```python
from build123d import *

# Parameters (mm, degrees)
SKETCH1_W                     = 42
SKETCH1_H                     = 20
BOSS_EXTRUDE1_DEPTH           = 5
SKETCH2_W                     = 21.9
SKETCH2_H                     = 10
BOSS_EXTRUDE2_DEPTH           = 5
CBORE_FOR_M3_SHCS1_AT_2_COUNT = 2
CBORE_FOR_M3_SHCS1_AT_2_PITCH = 20
FILLET1_R                     = 1


with BuildPart() as part:
    # Sketch1 → Boss-Extrude1 (new body)
    with BuildSketch(Plane(origin=(0, 0, 0), x_dir=(1, 0, 0), z_dir=(0, 1, 0))):
        Rectangle(SKETCH1_W, SKETCH1_H)
    extrude(amount=BOSS_EXTRUDE1_DEPTH)

    # Sketch2 → Boss-Extrude2 (add)
    with BuildSketch(Plane(origin=(0, 5, 0), x_dir=(1, 0, 0), z_dir=(0, 1, 0))):
        with Locations((-10.05, 15)):
            Rectangle(SKETCH2_W, SKETCH2_H)
    extrude(amount=-BOSS_EXTRUDE2_DEPTH)

    # Sketch7 → CBORE for M3 SHCS1 (revolve, cut)
    with BuildSketch(Plane(origin=(-3.575, 5, -15), x_dir=(0, 0, 1), z_dir=(1, 0, 0))):
        Polygon((0, 0), (0, 5), (1.7, 5), (1.7, 3), (3.25, 3), (3.25, 0.020977491), (3.275, 0), align=None)
    cbore_for_m3_shcs1 = revolve(axis=Axis((-3.575, 11.35, -15), (0, -1, 0)), mode=Mode.SUBTRACT)

    # CBORE for M3 SHCS1 at 2: CBORE for M3 SHCS1 ×2
    with Locations(*[(0, 0, i * CBORE_FOR_M3_SHCS1_AT_2_PITCH) for i in range(1, CBORE_FOR_M3_SHCS1_AT_2_COUNT)]):
        add(cbore_for_m3_shcs1, mode=Mode.SUBTRACT)

    # Fillet1
    fillet1_edges = [part.edges().sort_by_distance(p)[0] for p in [
        (-21, 2.5, -20),
        (0.9, 2.5, -20),
        (21, 2.5, -10),
        (21, 2.5, 10),
        (-21, 2.5, 10),
    ]]
    fillet(fillet1_edges, radius=FILLET1_R)


solid = part.part
```
Could you check a few things on this model? Use its own coordinates, in mm. A direction names the side the tool comes from. Round coordinates to 2 decimals unless told otherwise and drop trailing zeros. Order: outer loops, then holes, each group sorted by start corner. A loop starts at its lowest first (then second) coordinate and runs counter-clockwise, first axis right, second up. Notation, with made-up numbers: M 0.25,87 L 31.25,87 A24 ccw 31.25,111 Z; hole C 85,-2 d4. An arc over 180 degrees is marked long. One line per question, with ' | ' between items. Start each with the question number.
(1) For P1, Ø3, axis at x = 11, y = 0.5, coming from the -Z side; P2, Ø10.5, axis at x = -3.575, z = 5, coming from the -Y side; P3, Ø4, axis at x = -3.575, z = 5, coming from the +Y side; P4, Ø3, axis at x = -3.575, z = -15, coming from the +Y side, each with a flat end and sliding along its axis, tell me the tip position at first contact or that it passes through.
(2) Suppose I cut it at A-A on z = -15. List the corners of the cut face in (x, y) for me (3 decimals), then the cut area to 3 significant figures.
(3) Please list where these lines run through material, in increasing order: line 1 along X through (y, z) = (4.3, 5) (3 decimals); line 2 along X through (y, z) = (1.55, 5) (3 decimals); line 3 along Z through (x, y) = (13, 1.8).
(4) Suppose I cut it at C-C on z = 5. List the corners of the cut face in (x, y) for me (3 decimals).
(5) Thinking about a two-plate mould opening in Z: for faces 4 (the face through (20.715, 2.535, -9.699)), 5 (the face through (-5.01, 1.01, 5.91)), 6 (the face through (-4.09, 1.01, -13.38)), 7 (the face through (0, 2, 10)), which applies, +Z half, -Z half, draft (parallel to the pull), parting line (faces both ways), or undercut?
(6) Suppose I cut it at B-B on y = 2.6. List the corners of the cut face in (x, z) for me (3 decimals).
(7) For faces 1 (the face through (-0.69, 3.51, 6.5)), 2 (the face through (10, 2, -10)), 3 (the face through (20.699, 2.535, 9.715)), which set-ups out of +Z, -Z, +X, -X, +Y, -Y let a thin tool reach every point of the face, with its end or its side?
(8) Suppose I cut it at D-D on x = 12. List the corners of the cut face in (y, z) for me.
Geometry results:
1) P1: z = -10 | P2: y = 0 | P3: y = 2 | P4: through
2) outline: M -21,0 L -5.275,0 L -5.275,2 L -6.825,2 L -6.825,4.979 L -6.85,5 L -21,5 Z; M -1.875,0 L 0.9,0 L 0.9,5 L -0.3,5 L -0.325,4.979 L -0.325,2 L -1.875,2 Z | area: 83.2 mm²
3) line 1: -21 to -6.825, -0.325 to 21 | line 2: -21 to -5.275, -1.875 to 21 | line 3: -10 to 10
4) outline: M -21,0 L -5.275,0 L -5.275,2 L -6.825,2 L -6.825,4.979 L -6.85,5 L -21,5 Z; M -1.875,0 L 21,0 L 21,5 L -0.3,5 L -0.325,4.979 L -0.325,2 L -1.875,2 Z
5) face 4: -Z half | face 5: undercut | face 6: undercut | face 7: +Z half
6) outline: M -21,-19 A1 ccw -20,-20 L -0.1,-20 A1 ccw 0.9,-19 L 0.9,-10 L 20,-10 A1 ccw 21,-9 L 21,9 A1 ccw 20,10 L -20,10 A1 ccw -21,9 Z; hole C -3.575,-15 d6.5; hole C -3.575,5 d6.5
7) face 1: +Y | face 2: -Z, +X, +Y, -Y | face 3: +Z, +X, +Y, -Y
8) outline: M 0,-10 L 5,-10 L 5,10 L 0,10 Z
